Geometry: final body of the model. Coordinates: model frame, mm. Face numbers are marked on the shaded views. A direction names the side the tool comes from. Coordinates: 2 decimals unless noted, no trailing zeros. Order: outer loops, then holes, each group sorted by start corner. A loop starts at its lowest first (then second) coordinate and runs counter-clockwise, first axis right, second up. Notation, with made-up numbers: (-25, 33.5) -> (-9, 33.5) arc R23 ccw to (-9, 50.5) -> close; hole circle Ø4 at (45.5, -10.5). An arc over 180 degrees is marked (long way). Use one line per item in the form item = value.
Autodesk Inventor part; units mm, degrees
ref_plane "YZ Plane" through (0, 0, 0) normal (1, 0, 0) x (0, 1, 0)
ref_plane "XZ Plane" through (0, 0, 0) normal (0, 1, 0) x (-1, 0, 0)
ref_plane "XY Plane" through (0, 0, 0) normal (0, 0, 1) x (1, 0, 0)
sketch "Sketch1" plane through (0, 0, 0) normal (0, 0, 1) x (1, 0, 0)
  line L0 (0, 0) -> (0, 76.2)
  line L1 (0, 76.2) -> (-25.4, 76.2)
  line L2 (-25.4, 76.2) -> (-25.4, 0)
  line L3 (-25.4, 0) -> (0, 0)
  dimension "d0" = 76.2
  dimension "d2" = 25.4
extrude "Extrusion1" add sketch "Sketch1" along normal blind 2.54
sketch "Sketch2" plane through (0, 0, 2.54) normal (0, 0, 1) x (1, 0, 0)
  line L0 (-25.4, 0) -> (-25.4, 2.54)
  line L1 (-25.4, 76.2) -> (-25.4, 0)
  line L2 (-25.4, 2.54) -> (0, 2.54)
  line L3 (0, 0) -> (0, 76.2)
  line L4 (0, 0) -> (-25.4, 0)
  line L5 (-25.4, 0) -> (0, 0)
  dimension "d5" = 2.54
extrude "Extrusion2" add sketch "Sketch2" along normal blind 76.2
hole "Hole1" at (-12.7, 2.54, 12.7) direction (0, -1, 0) diameter 6.35 end through all
pattern_linear "Rectangular Pattern1" count 3 spacing 25.4 along (0, 0, 1) of "Hole1"
hole "Hole2" at (-12.7, 12.7, 2.54) direction (0, 0, -1) diameter 6.35 end through all
pattern_linear "Rectangular Pattern2" count 3 spacing 25.4 along (0, 1, 0) of "Hole2"
properties part number "L-Gusset long"
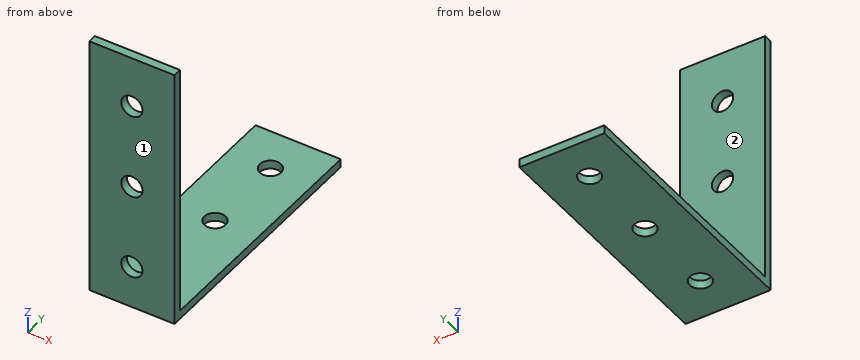
1) Section D-D, the plane x = -6.25. Output: boundary loops of the cut face in (y, z).
Results found:
outline = (0, 0) -> (76.2, 0) -> (76.2, 2.54) -> (2.54, 2.54) -> (2.54, 78.74) -> (0, 78.74) -> close
2) Material intervals for probe 1 along Z at (x, y) = (-12.7, 0.9) (3 decimals); probe 2 along Y at (x, z) = (-12.7, 2) (3 decimals); probe 3 along X at (y, z) = (1, 38), sorted ascending. Write a range as from..to.
Results found:
probe_1 = 0..9.525, 15.875..34.925, 41.275..60.325, 66.675..78.74
probe_2 = 0..9.525, 15.875..34.925, 41.275..60.325, 66.675..76.2
probe_3 = -25.4..-15.87, -9.53..0
3) Section A-A, the plane y = 12.7. Output: boundary loops of the cut face in (x, z) (3 decimals), and give its area (3 significant figures).
Results found:
outline = (-25.4, 0) -> (-15.875, 0) -> (-15.875, 2.54) -> (-25.4, 2.54) -> close; (-9.525, 0) -> (0, 0) -> (0, 2.54) -> (-9.525, 2.54) -> close
area = 48.4 mm2
4) Contact query for flat-ended pins moving along their axis: P1, Ø8.5, axis at x = -12.7, y = 63.5, coming from the -Z side; P2, Ø2, axis at x = -19.5, z = 47, coming from the +Y side; P3, Ø12.5, axis at x = -11, y = 43.5, coming from the +Z side. Output: stop coordinate, or through.
Results found:
P1 = 0
P2 = 2.54
P3 = 2.54
5) Section B-B, the plane x = -12.7. Give the number of separate pieces and of enclosed holes in the cut face, and give its area (3 significant figures).
Results found:
separate_pieces = 7
enclosed_holes = 0
area = 290 mm2
6) Access query for the marked faces 1 and 2. Directions: +Z, -Z, +X, -X, +Y, -Y. A direction counts if a zero-diameter tool reaches every point of the face in a straight line with its end or side. Return the directions, or none.
Results found:
face_1 = +Z, -Z, +X, -X, -Y
face_2 = +Z, +X, -X, +Y
